Check sheet for the modelled part. Datum: model origin and axes. Units: mm. Face numbers are marked on the shaded views. A direction names the side the tool comes from. Coordinates: 2 decimals unless noted, no trailing zeros. Loops run counter-clockwise (first coordinate to the right, second up) from the corner with the lowest first, then second, coordinate; pieces in that order, holes last. Notation, with made-up numbers: (7.25, 72.25) - (64.25, 72.25) arc R18 ccw to (64.25, 79.25) - close; hole circle Ø7 at (88, 72). An arc over 180 degrees is marked (long way). Write each question's results on one line, items separated by ' | '. Start each with the question number.
1. Cross-section at D-D (x = 31). Record the cut outline in (y, z).
2. Cross-section at C-C (y = 5.25). Record the cut outline in (x, z), and give its area (3 significant figures).
3. Cross-section at A-A (x = 0). Record the cut outline in (y, z), and give its area (3 significant figures).
4. Thickness scan on line 1 (Z direction, x = 10, y = 1); line 2 (Y direction, x = 20.5, z = -1.5); line 3 (X direction, y = 3.5, z = -2.75). Record the ranges inside material, lowest first. Write a range as [from, to].
5. Cross-section at B-B (z = 0). Record the cut outline in (x, y), and give its area (3 significant figures).
6. Gauge pin test, flat ends, axial feed: P1, Ø0.8, axis at x = 30.5, y = 0, coming from the -Z side; P2, Ø2, axis at x = 44, z = 1, coming from the +Y side; P3, Ø2, axis at x = 56.04, y = 0, coming from the +Z side. Record the tip position at first contact, or that the pin passes through.
7. Tool access check on the marked faces 1, 2 and 3. Record the directions out of +Z, -Z, +X, -X, +Y, -Y that give a thin tool (end or side, any length) a straight path to the whole face; none if there is none.
```python
from build123d import *

# Parameters (mm, degrees)
SKETCH1_R           = 3.25
BOSS_EXTRUDE1_DEPTH = 1.5
SKETCH2_R           = 3
BOSS_EXTRUDE2_DEPTH = 6
SKETCH3_W           = 60
SKETCH3_H           = 3
BOSS_EXTRUDE3_DEPTH = 2.5
CHAMFER1_SIZE       = 4
CHAMFER1_SIZE2      = 40
SKETCH4_R           = 0.85
CUT_EXTRUDE1_DEPTH  = 0.5


with BuildPart() as part:
    # Sketch1 → Boss-Extrude1 (new body, symmetric)
    with BuildSketch(Plane(origin=(0, 0, 0), x_dir=(1, 0, 0), z_dir=(0, 1, 0))):
        Circle(SKETCH1_R)
    extrude(amount=BOSS_EXTRUDE1_DEPTH, both=True)

    # Sketch2 → Boss-Extrude2 (add, symmetric)
    with BuildSketch(Plane(origin=(0, 0, 0), x_dir=(1, 0, 0), z_dir=(0, 1, 0))):
        Circle(SKETCH2_R)
    extrude(amount=BOSS_EXTRUDE2_DEPTH, both=True)

    # Sketch3 → Boss-Extrude3 (add, symmetric)
    with BuildSketch(Plane.XY):
        with Locations((30, 0)):
            Rectangle(SKETCH3_W, SKETCH3_H)
    extrude(amount=BOSS_EXTRUDE3_DEPTH, both=True)

    # Chamfer1
    chamfer1_edges = [part.edges().sort_by_distance(p)[0] for p in [
        (60, 0, 2.5),
    ]]
    chamfer1_side = [part.faces().sort_by_distance(p)[0] for p in [
        (60, 0, 0),
    ]]
    chamfer(chamfer1_edges, length=CHAMFER1_SIZE, length2=CHAMFER1_SIZE2, reference=chamfer1_side[0])

    # Sketch4 → Cut-Extrude1 (cut)
    with BuildSketch(Plane(origin=(0, 0, -2.5), x_dir=(-1, 0, 0), z_dir=(0, 0, -1))):
        with Locations((-6.044728096, 0)):
            Circle(SKETCH4_R)
        with Locations((-11.044728096, 0)):
            Circle(SKETCH4_R)
        with Locations((-16.044728096, 0)):
            Circle(SKETCH4_R)
        with Locations((-21.044728096, 0)):
            Circle(SKETCH4_R)
        with Locations((-26.044728096, 0)):
            Circle(SKETCH4_R)
        with Locations((-31.044728096, 0)):
            Circle(SKETCH4_R)
        with Locations((-36.044728096, 0)):
            Circle(SKETCH4_R)
        with Locations((-41.044728096, 0)):
            Circle(SKETCH4_R)
        with Locations((-46.044728096, 0)):
            Circle(SKETCH4_R)
        with Locations((-51.044728096, 0)):
            Circle(SKETCH4_R)
        with Locations((-56.044728096, 0)):
            Circle(SKETCH4_R)
    extrude(amount=-CUT_EXTRUDE1_DEPTH, mode=Mode.SUBTRACT)


solid = part.part
```
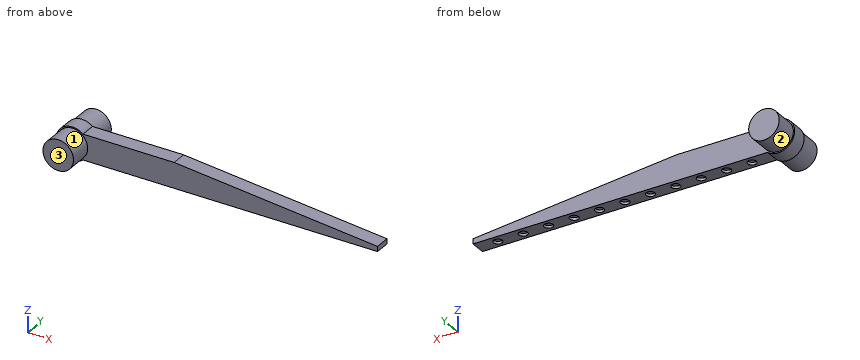
Established:
1) outline: (-1.5, -2.5) - (-0.85, -2.5) - (-0.85, -2) - (0.85, -2) - (0.85, -2.5) - (1.5, -2.5) - (1.5, 1.4) - (-1.5, 1.4) - close
2) outline: circle Ø6 at (0, 0) | area: 28.3 mm^2
3) outline: (-6, -3) - (-1.5, -3) - (-1.5, -3.25) - (1.5, -3.25) - (1.5, -3) - (6, -3) - (6, 3) - (1.5, 3) - (1.5, 3.25) - (-1.5, 3.25) - (-1.5, 3) - (-6, 3) - close | area: 73.5 mm^2
4) line 1: [-2.5, 2.5] | line 2: [-1.5, 1.5] | line 3: [-1.2, 1.2]
5) outline: (-3.25, -1.5) - (-3, -1.5) - (-3, -6) - (3, -6) - (3, -1.5) - (45, -1.5) - (45, 1.5) - (3, 1.5) - (3, 6) - (-3, 6) - (-3, 1.5) - (-3.25, 1.5) - close | area: 199 mm^2
6) P1: z = -2.5 | P2: y = 1.5 | P3: z = -1
7) face 1: -Y | face 2: +Y | face 3: +Z, -Z, +X, -X, -Y
